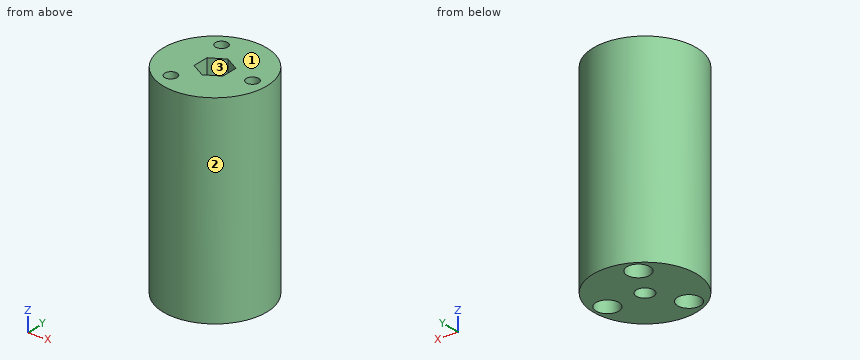
```python
from build123d import *

# Parameters (mm, degrees)
F0_R     = 18
F0_R_2   = 3
F1_DEPTH = 70
F2_R     = 3
F3_DEPTH = 64
F4_D     = 4.3
F5_D     = 8
F5_DEPTH = 65
F5_TIP   = 2.4034424761


with BuildPart() as f1:
    # F0 (on Top) → F1 (new body)
    with BuildSketch(Plane.XY):
        Circle(F0_R)
        Circle(F0_R_2, mode=Mode.SUBTRACT)
    extrude(amount=F1_DEPTH)

    # F2 (on face) → F3 (cut)
    with BuildSketch(Plane.XY.offset(70)):
        Polygon((5, -2.8867513459), (5, 2.8867513459), (0, 5.7735026919), (-5, 2.8867513459), (-5, -2.8867513459), (0, -5.7735026919), align=None)
        Circle(F2_R, mode=Mode.SUBTRACT)
    extrude(amount=-F3_DEPTH, mode=Mode.SUBTRACT)

    # F4 (through all)
    with Locations(Plane(origin=(0, 0, 0), x_dir=(1, 0, 0), z_dir=(0, 0, -1))):
        with Locations((13, 0), (-6.5, -11.2583302492), (-6.5, 11.2583302492)):
            Hole(F4_D / 2)

    # F5
    with Locations(Plane(origin=(0, 0, 0), x_dir=(1, 0, 0), z_dir=(0, 0, -1))):
        with Locations((13, 0), (-6.5, -11.2583302492), (-6.5, 11.2583302492)):
            Hole(F5_D / 2, depth=F5_DEPTH)
            with Locations((0, 0, -(F5_DEPTH + F5_TIP / 2))):  # 118° drill point
                Cone(0, F5_D / 2, F5_TIP, mode=Mode.SUBTRACT)


solid = f1.part
```
Geometry check sheet. Reference: the model listing, model coordinates, mm. Face numbers are marked on the shaded views. Coordinates: 2 decimals unless noted, no trailing zeros. Order: outer loops, then holes, each group sorted by start corner. A loop starts at its lowest first (then second) coordinate and runs counter-clockwise, first axis right, second up.
Item 1: Mould release check, pull along Y, two halves, no side actions. Record for the marked faces 1, 2 and 3: released by +Y, released by -Y, zero draft, split by the parting line, or undercut.
Item 2: Section check C-C (z = 58). Enter the section's corners in (x, y), plus the area to 3 significant figures.
Item 3: Section check D-D (x = -6.5). Enter the section's corners in (y, z), plus the area to 3 significant figures.
Item 4: Section check A-A (y = 0). Enter the section's corners in (x, z).
Item 5: Scan lines: line 1 along Y through (x, z) = (0, 3.2); line 2 along Y through (x, z) = (-7, 38.5); line 3 along Y through (x, z) = (-6.5, 50). Record each from-to range of solid material in increasing order.
Item 6: Depth check by flat-ended pin: pin 1 (12 mm diameter, centred on x = 5.5, z = 31.5, fed in from -Y); pin 2 (10 mm diameter, centred on x = -7, z = 34, fed in from +Y); pin 3 (9 mm diameter, centred on x = 13, y = 0, fed in from +Z); pin 4 (1.5 mm diameter, centred on x = 13.5, y = 2.5, fed in from -Z). Enter the tip coordinate at first touch or a pass-through.
Item 7: Section check B-B (x = 13). Enter the section's corners in (y, z), plus the area to 3 significant figures.
Check sheet entries:
1. face 1: zero draft
1. face 2: split by the parting line
1. face 3: undercut
2. outline: circle Ø36 at (0, 0); hole circle Ø8 at (-6.5, -11.26); hole circle Ø8 at (-6.5, 11.26); hole (-5, -2.89) - (0, -5.77) - (5, -2.89) - (5, 2.89) - (0, 5.77) - (-5, 2.89) - close; hole circle Ø8 at (13, 0)
2. area: 780 mm2
3. outline: (-16.79, 0) - (-15.26, 0) - (-15.26, 65) - (-13.41, 66.11) - (-13.41, 70) - (-16.79, 70) - close; (-9.11, 66.11) - (-7.26, 65) - (-7.26, 0) - (7.26, 0) - (7.26, 65) - (9.11, 66.11) - (9.11, 70) - (-9.11, 70) - close; (13.41, 66.11) - (15.26, 65) - (15.26, 0) - (16.79, 0) - (16.79, 70) - (13.41, 70) - close
3. area: 1,260 mm2
4. outline: (-18, 0) - (-3, 0) - (-3, 6) - (-5, 6) - (-5, 70) - (-18, 70) - close; (3, 0) - (9, 0) - (9, 65) - (10.85, 66.11) - (10.85, 70) - (5, 70) - (5, 6) - (3, 6) - close; (15.15, 66.11) - (17, 65) - (17, 0) - (18, 0) - (18, 70) - (15.15, 70) - close
5. line 1: y = -18 to -3, 3 to 18
5. line 2: y = -16.58 to -15.23, -7.29 to 7.29, 15.23 to 16.58
5. line 3: y = -16.79 to -15.26, -7.26 to 7.26, 15.26 to 16.79
6. pin 1: stops at y = -18
6. pin 2: stops at y = 17.89
6. pin 3: stops at z = 70
6. pin 4: stops at z = 65.42
7. outline: (-12.45, 0) - (-4, 0) - (-4, 65) - (-2.15, 66.11) - (-2.15, 70) - (-12.45, 70) - close; (2.15, 66.11) - (4, 65) - (4, 0) - (12.45, 0) - (12.45, 70) - (2.15, 70) - close
7. area: 1,200 mm2
